Model file for the job. Use its own axes, mm. A direction names the side the tool comes from. Give positions to 0.01 mm unless a question says otherwise; leave off trailing zeros. Loops run counter-clockwise (first coordinate to the right, second up) from the corner with the lowest first, then second, coordinate; pieces in that order, holes last. Notation, with made-up numbers: (-38.75, -27) -> (-13.75, -27) arc R13 cw to (-13.75, -9) -> close; hole circle Ø10 at (55.5, 63.5). An arc over 180 degrees is marked (long way). Use CSV: the item, a comma, the result in double quotes. Start each with the question number.
(1) Flat gauge pins, fed straight in: pin 1 (1 mm diameter, centred on y = -21, z = -2.5, fed in from -X); pin 2 (1.5 mm diameter, centred on y = -26, z = -5.5, fed in from -X); pin 3 (3 mm diameter, centred on y = -6.5, z = -6, fed in from -X); pin 4 (2 mm diameter, centred on y = -6.5, z = 8.5, fed in from -X). Where does each tip first touch, or does it go through?
(2) Cut at A-A on y = -8. Write the cut outline in (x, z).
(3) 3-axis set-ups, long thin cutter, end or side, ignore diameter. For faces 1 (the conical face through (-0.132, 9.798, -9.849)), 2 (the flat face through (-4, 0, 5)): which of +Z, -Z, +X, -X, +Y, -Y reach the whole face in a straight line?
(4) Drill centre lines: probe 1 along Z at (x, y) = (0.25, -10.5); probe 2 along Z at (x, y) = (2.75, -22.5); probe 3 along Y at (x, z) = (-6.5, -2.5). Where is each one in solid material? Low to high.
from build123d import *

# Parameters (mm, degrees)
SKETCH2_R           = 6
BOSS_EXTRUDE1_DEPTH = 52
BOSS_EXTRUDE2_DEPTH = 10
SKETCH5_OUTSIDE_W   = 69.512
SKETCH5_OUTSIDE_H   = 72.278
SKETCH5_OUTSIDE_R   = 9.5
CUT_EXTRUDE1_DEPTH  = 10
CUT_EXTRUDE1_DRAFT  = -60
CHAMFER1_SIZE       = 1


with BuildPart() as part:
    # Sketch2 → Boss-Extrude1 (new body)
    with BuildSketch(Plane(origin=(0, 0, 0), x_dir=(1, 0, 0), z_dir=(0, 1, 0))):
        with Locations(Location((0, 0, 0), (0, 0, 270))):
            Circle(SKETCH2_R)
    extrude(amount=-BOSS_EXTRUDE1_DEPTH)

    # Sketch3 → Boss-Extrude2 (add)
    with BuildSketch(Plane(origin=(0, 0, 0), x_dir=(1, 0, 0), z_dir=(0, 1, 0))):
        Polygon((9.585446106, -5.334093763), (9.412183758, 5.634192953), (-0.173262348, 10.968286716), (-9.585446106, 5.334093763), (-9.412183758, -5.634192953), (0.173262348, -10.968286716), align=None)
    extrude(amount=BOSS_EXTRUDE2_DEPTH)


with BuildPart() as cut_extrude1_tool:
    # Sketch5 outside → Cut-Extrude1 (with draft: the straight prism first)
    with BuildSketch(Plane(origin=(0, 10, 0), x_dir=(1, 0, 0), z_dir=(0, 1, 0))):
        Rectangle(SKETCH5_OUTSIDE_W, SKETCH5_OUTSIDE_H)
        Circle(SKETCH5_OUTSIDE_R, mode=Mode.SUBTRACT)
    extrude(amount=-CUT_EXTRUDE1_DEPTH)
    # Cut-Extrude1: the draft: its side faces are tilted about the plane it starts from
    cut_extrude1_sides = [cut_extrude1_tool.faces().sort_by_distance(p)[0] for p in [
        (0, 5, 36.139),
        (34.756, 5, 0),
        (0, 5, -36.139),
        (-34.756, 5, 0),
        (-9.5, 5, 0),
    ]]
    draft(cut_extrude1_sides, Plane(origin=(0, 10, 0), x_dir=(1, 0, 0), z_dir=(0, 1, 0)), CUT_EXTRUDE1_DRAFT)


with BuildPart() as part_1:
    add(part.part)

    # Cut-Extrude1: cut by cut_extrude1_tool
    add(cut_extrude1_tool.part, mode=Mode.SUBTRACT)

    # Chamfer1
    chamfer1_edges = [part_1.edges().sort_by_distance(p)[0] for p in [
        (0, -52, -6),
    ]]
    chamfer(chamfer1_edges, length=CHAMFER1_SIZE)


solid = part_1.part
Check result:
1,pin 1,"x = -5.66"
1,pin 2,"x = -3.67"
1,pin 3,"x = -3.97"
1,pin 4,"through"
2,outline,"circle Ø12 at (0, 0)"
3,face 1,"-Z, +Y"
3,face 2,"-Y"
4,probe 1,"-5.99 to 5.99"
4,probe 2,"-5.33 to 5.33"
4,probe 3,"0 to 10"
